Part model, mm, in its own coordinate system. Round coordinates to 2 decimals unless told otherwise and drop trailing zeros. Order: outer loops, then holes, each group sorted by start corner. A loop starts at its lowest first (then second) coordinate and runs counter-clockwise, first axis right, second up. Notation, with made-up numbers: (65, -36.5) -> (119, -36.5) arc R19 ccw to (119, -26.5) -> close; hole circle Ø9 at (17, 32). An arc over 180 degrees is marked (long way). Use CSV: the item, a comma, the result in double quotes.
```python
from build123d import *

# Parameters (mm, degrees)
SKETCH_W               = 140
SKETCH_H               = 75
PAD_DEPTH              = 10
SKETCH001_W            = 40
SKETCH001_H            = 10
PAD001_DEPTH           = 95
SKETCH002_R            = 2.75
HOLE_DEPTH             = 10.001
LINEARPATTERN_COUNT    = 4
LINEARPATTERN_PITCH    = 28
SKETCH003_R            = 2.75
HOLE001_DEPTH          = 10.001
LINEARPATTERN001_COUNT = 2
LINEARPATTERN001_PITCH = 22
LINEARPATTERN002_COUNT = 2
LINEARPATTERN002_PITCH = 40
SKETCH004_R            = 2.75
HOLE002_DEPTH          = 10.001


with BuildPart() as part:
    # Sketch → Pad (new body)
    with BuildSketch(Plane.XY):
        with Locations((70, 37.5)):
            Rectangle(SKETCH_W, SKETCH_H)
    extrude(amount=PAD_DEPTH)

    # Sketch001 (on Face3 of Pad) → Pad001 (join)
    with BuildSketch(Plane(origin=(0, 75, 0), x_dir=(-1, 0, 0), z_dir=(0, 1, 0))):
        with Locations((-70, 5)):
            Rectangle(SKETCH001_W, SKETCH001_H)
    extrude(amount=PAD001_DEPTH)

    # Sketch002 (on Face5 of Pad001) → Hole (cut, through all)
    with BuildSketch(Plane.XY.offset(10)):
        with Locations((28, 5)):
            Circle(SKETCH002_R)
    hole = extrude(amount=-HOLE_DEPTH, mode=Mode.SUBTRACT)

    # LinearPattern: Hole ×4
    with Locations(*[(i * LINEARPATTERN_PITCH, 0, 0) for i in range(1, LINEARPATTERN_COUNT)]):
        add(hole, mode=Mode.SUBTRACT)

    # Sketch003 (on Face13 of LinearPattern) → Hole001 (cut, through all)
    with BuildSketch(Plane.XY.offset(10)):
        with Locations((59, 114.5)):
            Circle(SKETCH003_R)
    hole001 = extrude(amount=-HOLE001_DEPTH, mode=Mode.SUBTRACT)

    # LinearPattern001: Hole001 ×2
    with Locations(*[(i * LINEARPATTERN001_PITCH, 0, 0) for i in range(1, LINEARPATTERN001_COUNT)]):
        add(hole001, mode=Mode.SUBTRACT)

    # LinearPattern002: Hole001 ×2
    with Locations(*[(0, i * LINEARPATTERN002_PITCH, 0) for i in range(1, LINEARPATTERN002_COUNT)]):
        add(hole001, mode=Mode.SUBTRACT)

    # Sketch004 (on Face13 of LinearPattern002) → Hole002 (cut, through all)
    with BuildSketch(Plane.XY.offset(10)):
        with Locations((81, 154.5)):
            Circle(SKETCH004_R)
    extrude(amount=-HOLE002_DEPTH, mode=Mode.SUBTRACT)


solid = part.part
```
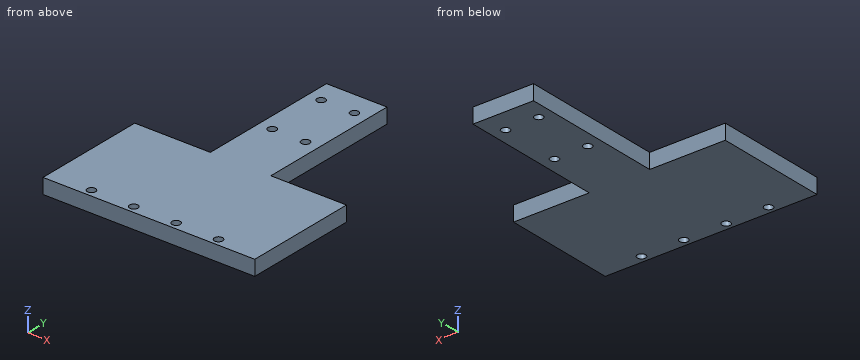
(1) Cut at C-C, the plane z = 5.75. State how many separate pieces and enclosed holes the cut face has, then the cut area to 3 significant figures.
Reply:
separate pieces,"1"
enclosed holes,"8"
area,"14,100 mm2"
(2) Probe probe 1 along Y at (x, z) = (59, 7.5); probe 2 along Y at (x, z) = (83, 2.25); probe 3 along Y at (x, z) = (112, 5.25). List the from-to ranges inside material, lowest first. Write a range as [from, to].
Reply:
probe 1,"[0, 111.75], [117.25, 151.75], [157.25, 170]"
probe 2,"[0, 2.44], [7.56, 112.61], [116.39, 152.61], [156.39, 170]"
probe 3,"[0, 2.25], [7.75, 75]"
(3) Drop flat-ended pins along their axis: P1, Ø7, axis at x = 112, y = 5, coming from the +Z side; P2, Ø3, axis at y = 132, z = 4.5, coming from the +X side; P3, Ø5, axis at x = 114, z = 7, coming from the +Y side; P4, Ø3, axis at y = 146, z = 4, coming from the -X side. Give the stop position or say it passes through.
Reply:
P1,"z = 10"
P2,"x = 90"
P3,"y = 75"
P4,"x = 50"
(4) Cut at D-D, the plane x = 37. Give the cut face in (y, z).
Reply:
outline,"(0, 0) -> (75, 0) -> (75, 10) -> (0, 10) -> close"
(5) Cut at A-A, the plane x = 112. Give the cut face in (y, z).
Reply:
outline,"(0, 0) -> (2.25, 0) -> (2.25, 10) -> (0, 10) -> close; (7.75, 0) -> (75, 0) -> (75, 10) -> (7.75, 10) -> close"
(6) Cut at B-B, the plane y = 5. Give the cut face in (x, z), then the cut area to 3 significant figures.
Reply:
outline,"(0, 0) -> (25.25, 0) -> (25.25, 10) -> (0, 10) -> close; (30.75, 0) -> (53.25, 0) -> (53.25, 10) -> (30.75, 10) -> close; (58.75, 0) -> (81.25, 0) -> (81.25, 10) -> (58.75, 10) -> close; (86.75, 0) -> (109.25, 0) -> (109.25, 10) -> (86.75, 10) -> close; (114.75, 0) -> (140, 0) -> (140, 10) -> (114.75, 10) -> close"
area,"1,180 mm2"
